For this review, take the finished solid that the model builds, in its own axes (mm). A direction names the side the tool comes from. Give positions to 0.01 mm unless a question says otherwise; leave off trailing zeros. Write each loop counter-clockwise with the first axis right and the second up, starting at its lowest first coordinate (ties: lowest second). Pieces come first, ordered by that corner, then holes. Notation, with made-up numbers: M 47.25,29.5 L 102.25,29.5 A20 ccw 102.25,35.5 Z; hole C 20.25,57.5 d6. An arc over 180 degrees is marked long. Write item = value, one per line.
```python
from build123d import *

# Parameters (mm, degrees)
SKETCH002_R             = 2
POCKET_DEPTH            = 10.001
POCKET_DEPTH_BACK       = 12.001
SKETCH003_W             = 10
SKETCH003_H             = 3.516841
POCKET001_DEPTH         = 7.003075
POCKET001_DEPTH_BACK    = 7.003075
BODY001_PLACEMENT_ANGLE = 180


with BuildPart() as part:
    # Sketch001 → Revolution001 (revolve)
    with BuildSketch(Plane.XY):
        Polygon((0, -12), (-3.8, -12), (-3.8, 0), (-7.002075, 0), (0, 10), align=None)
    revolve(axis=Axis((0, 0, 0), (0, 1, 0)))

    # Sketch002 → Pocket (cut, two sides)
    with BuildSketch(Plane.XZ) as pocket_sk:
        Circle(SKETCH002_R)
    extrude(amount=-POCKET_DEPTH, mode=Mode.SUBTRACT)
    extrude(pocket_sk.sketch, amount=POCKET_DEPTH_BACK, mode=Mode.SUBTRACT)

    # Sketch003 → Pocket001 (cut, two sides)
    with BuildSketch(Plane.XY) as pocket001_sk:
        with Locations((0, 7.75842)):
            Rectangle(SKETCH003_W, SKETCH003_H)
    extrude(amount=-POCKET001_DEPTH, mode=Mode.SUBTRACT)
    extrude(pocket001_sk.sketch, amount=POCKET001_DEPTH_BACK, mode=Mode.SUBTRACT)


with BuildPart() as part_1:
    # Body001 placement: moved
    add(part.part.moved(Location((0, 15, 0))).rotate(Axis((0, 15, 0), (1, 0, 0)), BODY001_PLACEMENT_ANGLE))


solid = part_1.part
```
1. We need section B-B, the plane y = 17.5. Write out the cut boundary in (x, z).
Responses:
outline = C 0,0 d7.6; hole C 0,0 d4
2. Insertion check: P1, Ø6, axis at x = -3, y = 12, coming from the -Z side; P2, Ø5, axis at x = 0, z = 0, coming from the +Y side; P3, Ø2, axis at y = 14, z = 1, coming from the +X side; P4, Ø2, axis at x = -4.5, y = 13.5, coming from the +Z side. Each pin has a flat end and moves straight along its axis. Give the tip position at first contact, or say it passes through.
Responses:
P1 = -6.59
P2 = 27
P3 = 6.94
P4 = 5.22
3. We need section A-A, the plane x = 0. Write out the cut boundary in (y, z).
Responses:
outline = M 9,-2.8 L 15,-7 L 15,-3.8 L 27,-3.8 L 27,-2 L 9,-2 Z; M 9,2 L 27,2 L 27,3.8 L 15,3.8 L 15,7 L 9,2.8 Z
4. We need section C-C, the plane y = 12.5. Write out the cut boundary in (x, z).
Responses:
outline = C 0,0 d10.5; hole C 0,0 d4
5. For line 1 along Z through (x, y) = (0, 24); line 2 along X through (y, z) = (13, -1.75); line 3 along Z through (x, y) = (0.75, 21.25), list the stretches that pass through material, from the lowest coordinate up. Write a range as from..to.
Responses:
line_1 = -3.8..-2, 2..3.8
line_2 = -5.32..-0.97, 0.97..5.32
line_3 = -3.73..-1.85, 1.85..3.73
6. Machinability: for faces 1 (the face through (3, 15, 3)), 2 (the face through (-3.311, 9.958, -1.043)), which of the approach directions +Z, -Z, +X, -X, +Y, -Y give a long, thin tool a straight path to every point of the face, cutting with its end or side? Answer none if there is none.
Responses:
face_1 = +Y
face_2 = -Y
